Geometry check sheet. Reference: the model listing, model coordinates, mm. A direction names the side the tool comes from. Coordinates: 2 decimals unless noted, no trailing zeros. Write each loop counter-clockwise with the first axis right and the second up, starting at its lowest first coordinate (ties: lowest second). Pieces come first, ordered by that corner, then holes. Notation, with made-up numbers: (72.5, -16.75) -> (128.5, -16.75) arc R32 cw to (128.5, 15.25) -> close; hole circle Ø2 at (46, 11). An arc over 180 degrees is marked (long way). Put each result on its own line as item: value. Start each with the question number.
from build123d import *

# Parameters (mm, degrees)
F0_W     = 3.5634012893
F0_H     = 2.3720003664
F1_DEPTH = 5


with BuildPart() as f1:
    # F0 (on Front) → F1 (new body)
    with BuildSketch(Plane.XZ):
        with BuildLine():
            Line((-2, 0), (0, 0))
            add(Edge.make_bspline(
                [(0, 0), (-0.1836561132, 1.7094361829), (-0.1397413061, 9.7580692578), (2.5518890591, 1.2595293557), (2.3045632429, 0)],
                knots=[0, 0, 0, 0, 0.4944254575, 1, 1, 1, 1], degree=3))
            Line((2.3045632429, 0), (4.3045632429, 0))
            add(Edge.make_bspline(
                [(1.898295837, 5.931569832), (3.3228321005, 4.8468001157), (3.5423423469, 2.2009662159), (4.3045632429, 0)],
                knots=[0.627484657, 0.627484657, 0.627484657, 0.627484657, 1, 1, 1, 1], degree=3))
            add(Edge.make_bspline(
                [(-1.5685537924, 5.7355813877), (-0.8538090003, 6.6826607519), (0.8490885432, 6.7305303973), (1.898295837, 5.931569832)],
                knots=[0.3531176051, 0.3531176051, 0.3531176051, 0.3531176051, 0.627484657, 0.627484657, 0.627484657, 0.627484657], degree=3))
            add(Edge.make_bspline(
                [(-2, 0), (-1.77153203, 1.8082654117), (-2.4884491206, 4.5166653604), (-1.5685537924, 5.7355813877)],
                knots=[0, 0, 0, 0, 0.3531176051, 0.3531176051, 0.3531176051, 0.3531176051], degree=3))
        make_face()
        with BuildLine():
            add(Edge.make_bspline(
                [(-1.5685537924, 5.7355813877), (-2.1986037273, 7.3149230589), (-1.4040608509, 9.1362467506), (-5.3149314083, 8.6162903235), (-6.5138074569, 8.659985655)],
                knots=[0, 0, 0, 0, 0.1835397267, 0.372551207, 0.372551207, 0.372551207, 0.372551207], degree=3))
            add(Edge.make_bspline(
                [(-1.5685537924, 5.7355813877), (-0.8538090003, 6.6826607519), (0.8490885432, 6.7305303973), (1.898295837, 5.931569832)],
                knots=[0.3531176051, 0.3531176051, 0.3531176051, 0.3531176051, 0.627484657, 0.627484657, 0.627484657, 0.627484657], degree=3))
            add(Edge.make_bspline(
                [(1.9229257877, 6.4971952265), (1.9126104325, 6.3173946518), (1.903779138, 6.1289676696), (1.898295837, 5.931569832)],
                knots=[0.9801694628, 0.9801694628, 0.9801694628, 0.9801694628, 1, 1, 1, 1], degree=3))
            add(Edge.make_bspline(
                [(1.9229257877, 6.4971952265), (1.9141740763, 6.5088301842), (1.9156850526, 6.5277113359), (1.9261891554, 6.5529953329)],
                knots=[0.577436763, 0.577436763, 0.577436763, 0.577436763, 0.5928976619, 0.5928976619, 0.5928976619, 0.5928976619], degree=3))
            add(Edge.make_bspline(
                [(1.8293032252, 8.9529328765), (2.1069112235, 8.4276675068), (1.9918291417, 7.6549231128), (1.9261891554, 6.5529953329)],
                knots=[0.8553520328, 0.8553520328, 0.8553520328, 0.8553520328, 0.978107761, 0.978107761, 0.978107761, 0.978107761], degree=3))
            add(Edge.make_bspline(
                [(1.0782698656, 9.5595878301), (1.4596732733, 9.4110932651), (1.6923053765, 9.2121481228), (1.8293032252, 8.9529328765)],
                knots=[0.7947728319, 0.7947728319, 0.7947728319, 0.7947728319, 0.8553520328, 0.8553520328, 0.8553520328, 0.8553520328], degree=3))
            add(Edge.make_bspline(
                [(0.9437969367, 9.6078676818), (0.9904450196, 9.5924058566), (1.0353015402, 9.576317001), (1.0782698656, 9.5595878301)],
                knots=[0.7879480717, 0.7879480717, 0.7879480717, 0.7879480717, 0.7947728319, 0.7947728319, 0.7947728319, 0.7947728319], degree=3))
            ThreePointArc((0.9437969367, 9.6078676818), (-0.2678500801, 9.3925558637), (-1.3808027632, 9.9177072682))
            add(Edge.make_bspline(
                [(-6.5138074569, 9.4688323455), (-5.3055520235, 9.7611397753), (-3.1719225069, 9.9688662745), (-1.3808027632, 9.9177072682)],
                knots=[0.5439344229, 0.5439344229, 0.5439344229, 0.5439344229, 0.7049021627, 0.7049021627, 0.7049021627, 0.7049021627], degree=3))
            Line((-6.5138074569, 9.4688323455), (-6.5138074569, 8.659985655))
        make_face()
        with BuildLine():
            Line((-6.5138074569, 6.5773790702), (-6.5138074569, 8.659985655))
            add(Edge.make_bspline(
                [(-6.5138074569, 8.659985655), (-6.7281794928, 8.667798854), (-6.9174435476, 8.6854435894), (-7.0701856166, 8.7181232441)],
                knots=[0.372551207, 0.372551207, 0.372551207, 0.372551207, 0.4063485089, 0.4063485089, 0.4063485089, 0.4063485089], degree=3))
            Line((-7.0701856166, 8.7181232441), (-7.0701856166, 6.5773790702))
            Line((-7.0701856166, 6.5773790702), (-6.5138074569, 6.5773790702))
        make_face()
        with BuildLine():
            add(Edge.make_bspline(
                [(-6.5138074569, 8.659985655), (-6.7281794928, 8.667798854), (-6.9174435476, 8.6854435894), (-7.0701856166, 8.7181232441)],
                knots=[0.372551207, 0.372551207, 0.372551207, 0.372551207, 0.4063485089, 0.4063485089, 0.4063485089, 0.4063485089], degree=3))
            Line((-6.5138074569, 8.659985655), (-6.5138074569, 9.4688323455))
            add(Edge.make_bspline(
                [(-7.0701856166, 9.3033018375), (-6.9198476576, 9.360551064), (-6.7319027313, 9.416069604), (-6.5138074569, 9.4688323455)],
                knots=[0.5148790573, 0.5148790573, 0.5148790573, 0.5148790573, 0.5439344229, 0.5439344229, 0.5439344229, 0.5439344229], degree=3))
            Line((-7.0701856166, 9.3033018375), (-7.0701856166, 8.7181232441))
        make_face()
        with BuildLine():
            add(Edge.make_bspline(
                [(1.9229257877, 6.4971952265), (1.9141740763, 6.5088301842), (1.9156850526, 6.5277113359), (1.9261891554, 6.5529953329)],
                knots=[0.577436763, 0.577436763, 0.577436763, 0.577436763, 0.5928976619, 0.5928976619, 0.5928976619, 0.5928976619], degree=3))
            add(Edge.make_bspline(
                [(1.9261891554, 6.5529953329), (1.9250867215, 6.5344882817), (1.923998234, 6.5158883752), (1.9229257877, 6.4971952265)],
                knots=[0.978107761, 0.978107761, 0.978107761, 0.978107761, 0.9801694628, 0.9801694628, 0.9801694628, 0.9801694628], degree=3))
        make_face()
        with BuildLine():
            add(Edge.make_bspline(
                [(1.9261891554, 6.5529953329), (1.9250867215, 6.5344882817), (1.923998234, 6.5158883752), (1.9229257877, 6.4971952265)],
                knots=[0.978107761, 0.978107761, 0.978107761, 0.978107761, 0.9801694628, 0.9801694628, 0.9801694628, 0.9801694628], degree=3))
            add(Edge.make_bspline(
                [(1.0782698656, 9.5595878301), (4.0481531599, 10.0701912701), (9.609540077, 10.9247415729), (2.0872194249, 6.2787751448), (1.9229257877, 6.4971952265)],
                knots=[0, 0, 0, 0, 0.2871932674, 0.577436763, 0.577436763, 0.577436763, 0.577436763], degree=3))
            add(Edge.make_bspline(
                [(1.0782698656, 9.5595878301), (1.4596732733, 9.4110932651), (1.6923053765, 9.2121481228), (1.8293032252, 8.9529328765)],
                knots=[0.7947728319, 0.7947728319, 0.7947728319, 0.7947728319, 0.8553520328, 0.8553520328, 0.8553520328, 0.8553520328], degree=3))
            add(Edge.make_bspline(
                [(1.9261891554, 6.5529953329), (2.0726362175, 6.9055020769), (5.6506443881, 9.9217752461), (3.1918898004, 9.2252642405), (1.8293032252, 8.9529328765)],
                knots=[0.5928976619, 0.5928976619, 0.5928976619, 0.5928976619, 0.8084518359, 1, 1, 1, 1], degree=3))
        make_face()
        with BuildLine():
            add(Edge.make_bspline(
                [(-7.0701856166, 8.7181232441), (-7.0925674088, 8.7229119002), (-7.4335820034, 8.8036195657), (-7.6231094084, 9.0330063205), (-7.2271410881, 9.2435326388), (-7.0701856166, 9.3033018375)],
                knots=[0.4063485089, 0.4063485089, 0.4063485089, 0.4063485089, 0.4113009375, 0.4845447449, 0.5148790573, 0.5148790573, 0.5148790573, 0.5148790573], degree=3))
            Line((-7.0701856166, 8.7181232441), (-7.0701856166, 9.3033018375))
        make_face()
        with BuildLine():
            add(Edge.make_bspline(
                [(-7.0701856166, 9.3033018375), (-6.9198476576, 9.360551064), (-6.7319027313, 9.416069604), (-6.5138074569, 9.4688323455)],
                knots=[0.5148790573, 0.5148790573, 0.5148790573, 0.5148790573, 0.5439344229, 0.5439344229, 0.5439344229, 0.5439344229], degree=3))
            Line((-6.5138074569, 9.4688323455), (-6.5138074569, 10.958660394))
            Line((-6.5138074569, 10.958660394), (-6.5138074569, 13.3306607604))
            Line((-6.5138074569, 13.3306607604), (-7.0701856166, 13.3306607604))
            Line((-7.0701856166, 13.3306607604), (-7.0701856166, 9.3033018375))
        make_face()
        with BuildLine():
            ThreePointArc((2.0273415276, 11.4021254703), (-0.8095538544, 13.2608175444), (-1.3808027632, 9.9177072682))
            add(Edge.make_bspline(
                [(-1.3808027632, 9.9177072682), (-0.4567345775, 9.891313494), (0.376167847, 9.796012214), (0.9437969367, 9.6078676818)],
                knots=[0.7049021627, 0.7049021627, 0.7049021627, 0.7049021627, 0.7879480717, 0.7879480717, 0.7879480717, 0.7879480717], degree=3))
            ThreePointArc((0.9437969367, 9.6078676818), (1.7354412109, 10.3540999587), (2.0273415276, 11.4021254703))
        make_face()
        with BuildLine():
            add(Edge.make_bspline(
                [(-1.3808027632, 9.9177072682), (-0.4567345775, 9.891313494), (0.376167847, 9.796012214), (0.9437969367, 9.6078676818)],
                knots=[0.7049021627, 0.7049021627, 0.7049021627, 0.7049021627, 0.7879480717, 0.7879480717, 0.7879480717, 0.7879480717], degree=3))
            ThreePointArc((-1.3808027632, 9.9177072682), (-0.2678500801, 9.3925558637), (0.9437969367, 9.6078676818))
        make_face()
        with Locations((-4.7321068123, 12.1446605772)):
            Rectangle(F0_W, F0_H)
    extrude(amount=F1_DEPTH)


solid = f1.part
Item 1: Go/stop test with flat-tipped pins: P1, Ø2, axis at x = -3.5, y = -1.5, coming from the +Z side; P2, Ø1, axis at y = -2, z = 7, coming from the +X side; P3, Ø1.1, axis at y = -3.5, z = 7.5, coming from the -X side. Record where each tip stops, or that it passes through.
Item 2: Scan lines: line 1 along Z through (x, y) = (2.75, -3.6); line 2 along Z through (x, y) = (2.5, -3.6); line 3 along X through (y, z) = (-0.25, 7.25). Record each from-to range of solid material in increasing order. Write a range as [from, to].
Item 3: Section check B-B, the plane x = 3. Give the number of separate pieces and of enclosed holes in the cut face, and give its area (3 significant figures).
Item 4: Mould release check, pull along Z, two halves, no side actions. Record for faces 6 (the flat face through (-6.514, -2, 8)), 7 (the flat face through (-5, -2, 13.331)), 8 (the flat face through (-6.514, -2, 10)): released by +Z, released by -Z, zero draft, split by the parting line, or undercut.
Item 5: Access from +Z, -Z, +X, -X, +Y, -Y to the whole of each face (thin tool, end or side, straight path). Record for faces 1 (the flat face through (-7.07, -2, 8)), 2 (the flat face through (-5, -2, 10.959)), 3 (the flat face through (-2.95, -2, 12)), 4 (the flat face through (-7.07, -2, 11)), 5 (the flat face through (-1, 0, 8)).
Item 6: Section check A-A, the plane z = 12. Enter the section's corners in (x, y), and give its area (3 significant figures).
From the geometry:
1. P1: z = 13.33
1. P2: x = 3.88
1. P3: x = -7.07
2. line 1: [0, 4.89], [6.82, 7.46], [9.14, 9.84]
2. line 2: [0, 5.29], [6.69, 7.21], [9.09, 9.8]
2. line 3: [-7.07, -6.51], [-1.96, 1.97], [2.54, 3.48]
3. separate pieces: 3
3. enclosed holes: 0
3. area: 28.9 mm²
4. face 6: zero draft
4. face 7: released by +Z
4. face 8: undercut
5. face 1: -Z, -X, +Y, -Y
5. face 2: +Y, -Y
5. face 3: +Z, +Y, -Y
5. face 4: +Z, -X, +Y, -Y
5. face 5: +Z, -Z, +X, -X, +Y
6. outline: (-7.07, -5) -> (-2.95, -5) -> (-2.95, 0) -> (-7.07, 0) -> close; (-1.94, -5) -> (1.94, -5) -> (1.94, 0) -> (-1.94, 0) -> close
6. area: 40.0 mm²
